```python
from build123d import *

# Parameters (mm, degrees)
SKETCH1_W           = 7
SKETCH1_H           = 7
BOSS_EXTRUDE1_DEPTH = 3
CUT_EXTRUDE1_DEPTH  = 7
CUT_EXTRUDE2_DEPTH  = 11
SKETCH4_R           = 1.8
CUT_EXTRUDE3_DEPTH  = 0.8
CUT_EXTRUDE4_DEPTH  = 0.4


with BuildPart() as part:
    # Sketch1 → Boss-Extrude1 (new body)
    with BuildSketch(Plane(origin=(0, 0, 0), x_dir=(1, 0, 0), z_dir=(0, 1, 0))):
        with Locations((3.5, 3.5)):
            Rectangle(SKETCH1_W, SKETCH1_H)
    extrude(amount=BOSS_EXTRUDE1_DEPTH)

    # Sketch2 → Cut-Extrude1 (cut)
    with BuildSketch(Plane.XY):
        Polygon((0, 0), (0.7, 3), (0, 3), align=None)
        Polygon((7, 0), (6.3, 3), (7, 3), align=None)
    extrude(amount=-CUT_EXTRUDE1_DEPTH, mode=Mode.SUBTRACT)

    # Sketch3 → Cut-Extrude2 (cut)
    with BuildSketch(Plane(origin=(0, 0, 0), x_dir=(0, 0, -1), z_dir=(1, 0, 0))):
        Polygon((0, 0), (0.7, 3), (0, 3), align=None)
        Polygon((7, 3), (6.3, 3), (7, 0), align=None)
    extrude(amount=CUT_EXTRUDE2_DEPTH, mode=Mode.SUBTRACT)

    # Sketch4 → Cut-Extrude3 (cut)
    with BuildSketch(Plane.XZ):
        with Locations(Location((3.5, -3.5, 0), (0, 0, 270))):
            Circle(SKETCH4_R)
    extrude(amount=-CUT_EXTRUDE3_DEPTH, mode=Mode.SUBTRACT)

    # Sketch5 → Cut-Extrude4 (cut)
    with BuildSketch(Plane(origin=(0, 3, 0), x_dir=(1, 0, 0), z_dir=(0, 1, 0))):
        Polygon((3.236309529, 1.779523254), (3.236309529, 4.696189921), (2.204258247, 4.696189921), (2.204258247, 5.279523254), (4.941437734, 5.279523254), (4.941437734, 4.696189921), (3.909386452, 4.696189921), (3.909386452, 1.779523254), align=None)
    extrude(amount=-CUT_EXTRUDE4_DEPTH, mode=Mode.SUBTRACT)


solid = part.part
```
Geometry: final body of the model. Coordinates: model frame, mm. A direction names the side the tool comes from. Round coordinates to 2 decimals unless told otherwise and drop trailing zeros. Write each loop counter-clockwise with the first axis right and the second up, starting at its lowest first coordinate (ties: lowest second). Pieces come first, ordered by that corner, then holes. Notation, with made-up numbers: (-37, -7) -> (-9, -7) arc R27 ccw to (-9, 18) -> close; hole circle Ø11 at (-1.5, 31). An arc over 180 degrees is marked (long way). Use CSV: the item, a comma, the result in double quotes. Start each with the question number.
Q1. Reachability of faces 1 (the face through (2, 0, -5)), 2 (the face through (4, 0.8, -3)) from +Z, -Z, +X, -X, +Y, -Y: full face, straight path, thin tool, end or side. Return the list, or none.
Q2. First-contact query: pin 1 Ø3 at (x, z) = (3.5, -3.5) entering from -Y. Flat tip, straight axial feed; report the tip coordinate or a pass-through.
Q3. Section B-B (x = 3.5). Return loops of the section in (y, z).
Q4. Section C-C (y = 1.4). Return loops of the section in (x, z).
Q5. Line query: L1, parallel to Y at x = 4.5, z = -3; L2, parallel to X at y = 0.2, z = -3.5; L3, parallel to X at y = 0.65, z = -3.5. Output: solid intervals per line, ascending.
Q6. Section A-A (z = -3.5). Return loops of the section in (x, y), plus the area to 3 significant figures.
Q7. Pull-direction query (Z, two-part tool) for faces 3 (the face through (4.041, 0.394, -5.217)), 4 (the face through (0.345, 1.479, -3.451)), 5 (the face through (3.451, 1.479, -0.345)); classes: pulls with the +Z half, pulls with the -Z half, needs draft (parallel to the pull), parting line crosses it, or undercut.
Q8. Section D-D (x = 6). Return loops of the section in (y, z), plus the area to 3 significant figures.
Result sheet:
1,face 1,"+Z, -Z, +X, -X, -Y"
1,face 2,"-Y"
2,pin 1,"y = 0.8"
3,outline,"(0, -7) -> (3, -6.3) -> (3, -5.28) -> (2.6, -5.28) -> (2.6, -1.78) -> (3, -1.78) -> (3, -0.7) -> (0, 0) -> (0, -1.7) -> (0.8, -1.7) -> (0.8, -5.3) -> (0, -5.3) -> close"
4,outline,"(0.33, -6.67) -> (6.67, -6.67) -> (6.67, -0.33) -> (0.33, -0.33) -> close"
5,L1,"0.8 to 3"
5,L2,"0.05 to 1.7, 5.3 to 6.95"
5,L3,"0.15 to 1.7, 5.3 to 6.85"
6,outline,"(0, 0) -> (1.7, 0) -> (1.7, 0.8) -> (5.3, 0.8) -> (5.3, 0) -> (7, 0) -> (6.3, 3) -> (3.91, 3) -> (3.91, 2.6) -> (3.24, 2.6) -> (3.24, 3) -> (0.7, 3) -> close"
6,area,"15.8 mm²"
7,face 3,"undercut"
7,face 4,"needs draft"
7,face 5,"pulls with the +Z half"
8,outline,"(0, -7) -> (3, -6.3) -> (3, -0.7) -> (0, 0) -> close"
8,area,"18.9 mm²"
